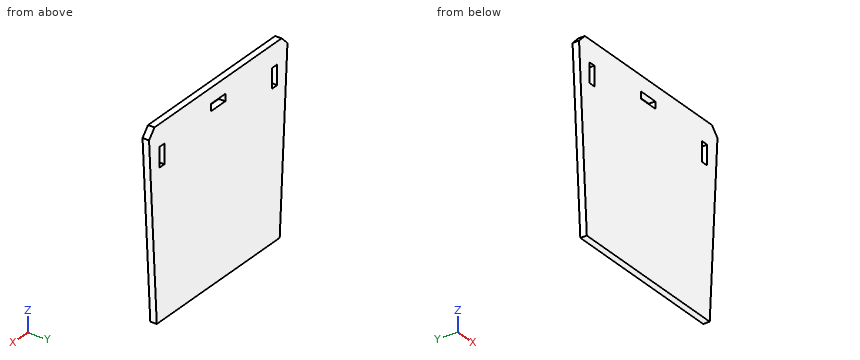
from build123d import *
from OCP.BRepFilletAPI import BRepFilletAPI_MakeChamfer

# Parameters (mm, degrees)
BOSS_EXTRUDE1_DEPTH = 15
CUT_EXTRUDE1_DEPTH  = 469.027776953
CHAMFER1_SIZE       = 20
CHAMFER1_SIZE2      = 18.885887556
SKETCH4_W           = 45.375817112
SKETCH4_H           = 15.979474245
CUT_EXTRUDE5_DEPTH  = 468.476442192


with BuildPart() as part:
    # Sketch1 → Boss-Extrude1 (new body)
    with BuildSketch(Plane(origin=(0, 0, 0), x_dir=(1, 0, 0), z_dir=(0, 1, 0))):
        Polygon((-225, -410.121933088), (-198.780229192, 20.01019046), (198.780229192, 20.01019046), (225, -410.121933088), align=None)
    extrude(amount=-BOSS_EXTRUDE1_DEPTH)

    # Sketch2 → Cut-Extrude1 (cut, through all)
    with BuildSketch(Plane.XZ.offset(15)):
        Polygon((190.662364216, 360.244932401), (190.758526229, 315.166919875), (174.389363372, 315.132000597), (174.293201359, 360.210013123), align=None)
    cut_extrude1 = extrude(amount=-CUT_EXTRUDE1_DEPTH, mode=Mode.SUBTRACT)

    # Mirror1: Cut-Extrude1 across plane
    add(cut_extrude1.mirror(Plane(origin=(0, 0, 0), x_dir=(0, 0, 1), z_dir=(1, 0, 0))), mode=Mode.SUBTRACT)

    # Chamfer1: one chamfer whose edges measure the first distance from different faces: ONE call of the kernel's chamfer builder (chamfer() names one face for all edges)
    chamfer1_edges_1 = [part.edges().sort_by_distance(p)[0] for p in [
        (-225, -7.5, 410.121933088),
    ]]
    chamfer1_side_1 = [part.faces().sort_by_distance(p)[0] for p in [
        (0, -7.5, 410.121933088),
    ]]
    chamfer1_edges_2 = [part.edges().sort_by_distance(p)[0] for p in [
        (225, -7.5, 410.121933088),
    ]]
    chamfer1_side_2 = [part.faces().sort_by_distance(p)[0] for p in [
        (211.890114596, -7.5, 195.055871314),
    ]]
    chamfer1 = BRepFilletAPI_MakeChamfer(part.part.solid().wrapped)
    for e in chamfer1_edges_1:
        chamfer1.Add(CHAMFER1_SIZE, CHAMFER1_SIZE2, e.wrapped, chamfer1_side_1[0].wrapped)  # the first distance lies on this face
    for e in chamfer1_edges_2:
        chamfer1.Add(CHAMFER1_SIZE, CHAMFER1_SIZE2, e.wrapped, chamfer1_side_2[0].wrapped)  # the first distance lies on this face
    add(Compound.cast(chamfer1.Shape()), mode=Mode.REPLACE)

    # Sketch4 → Cut-Extrude5 (cut, through all)
    with BuildSketch(Plane(origin=(0, 0, 0), x_dir=(1, 0, 0), z_dir=(0, 1, 0))):
        with Locations((0, -367.255161149)):
            Rectangle(SKETCH4_W, SKETCH4_H)
    extrude(amount=-CUT_EXTRUDE5_DEPTH, mode=Mode.SUBTRACT)


solid = part.part
Read the model definition and answer for the solid it produces. Units are mm, in the model's axes. Coordinates: 2 decimals unless noted, no trailing zeros. Write each loop counter-clockwise with the first axis right and the second up, starting at its lowest first coordinate (ties: lowest second). Pieces come first, ordered by that corner, then holes. Notation, with made-up numbers: M -29,59.5 L 14,59.5 A20 cw 14,93.5 Z; hole C 15.25,64.25 d10. An arc over 180 degrees is marked long. Use a Markdown table: item, result.
Q1. The part is cut by section B-B, the plane y = -5.5. Write down the section's boundary in (x, z), then the cut area to 3 significant figures.
Answer block:
| item | result |
|---|---|
| outline | M -223.85,391.27 L -198.78,-20.01 L 198.78,-20.01 L 223.78,390.16 L 206.11,410.12 L -205,410.12 Z; hole M -190.76,315.17 L -174.39,315.13 L -174.29,360.21 L -190.66,360.24 Z; hole M -22.69,359.27 L 22.69,359.27 L 22.69,375.24 L -22.69,375.24 Z; hole M 174.29,360.21 L 174.39,315.13 L 190.76,315.17 L 190.66,360.24 Z |
| area | 180,000 mm2 |
Q2. The part is cut by section D-D, the plane z = 143. Write down the section's boundary in (x, y), then the cut area to 3 significant figures.
Answer block:
| item | result |
|---|---|
| outline | M -208.72,-15 L 208.72,-15 L 208.72,0 L -208.72,0 Z |
| area | 6,260 mm2 |
Q3. Straight lines are drawn through the part: L1, parallel to Z at x = 12, y = -2.5; L2, parallel to X at y = -10, z = 337.5; L3, parallel to X at y = -1, z = 351. For each, find the intervals that lie inside material, in ascending order. Write a range as [from, to].
Answer block:
| item | result |
|---|---|
| L1 | z = [-20.01, 359.27], [375.24, 410.12] |
| L2 | x = [-220.57, -190.71], [-174.34, 174.34], [190.71, 220.57] |
| L3 | x = [-221.4, -190.68], [-174.31, 174.31], [190.68, 221.4] |
Q4. The part is cut by section A-A, the plane x = -1. Write down the section's boundary in (y, z), then the cut area to 3 significant figures.
Answer block:
| item | result |
|---|---|
| outline | M -15,-20.01 L 0,-20.01 L 0,359.27 L -15,359.27 Z; M -15,375.24 L 0,375.24 L 0,410.12 L -15,410.12 Z |
| area | 6,210 mm2 |
Q5. The part is cut by section C-C, the plane z = 11. Write down the section's boundary in (x, y), then the cut area to 3 significant figures.
Answer block:
| item | result |
|---|---|
| outline | M -200.67,-15 L 200.67,-15 L 200.67,0 L -200.67,0 Z |
| area | 6,020 mm2 |
Q6. This flat-tipped pin is pushed along its axis until it touches: pin 1 Ø4.5 at (y, z) = (-9, 367.5) entering from +X. Where does it stop, or does it pass through?
Answer block:
| item | result |
|---|---|
| pin 1 | stops at x = 222.54 |
